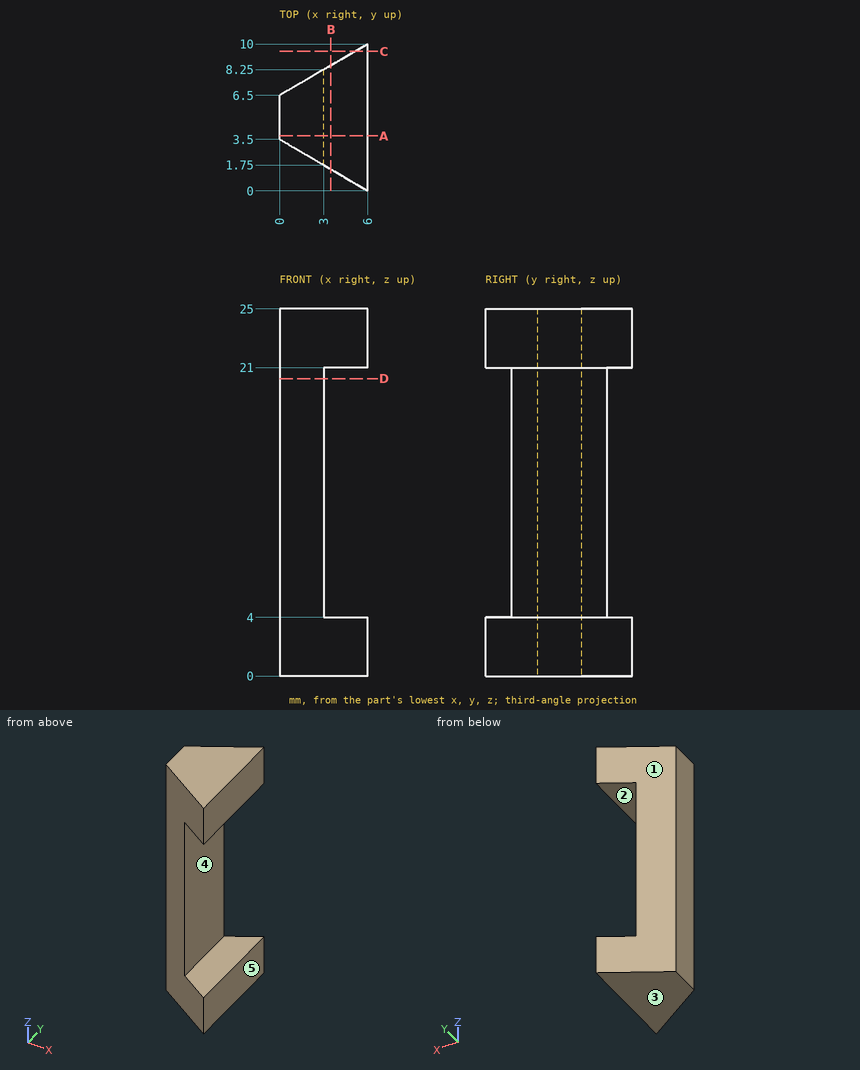
Input: dimensioned drawing with shaded views. Units: mm. Origin: part minimum x, y, z. A direction names the side the tool comes from. Give positions to 0.01 mm unless a question says otherwise; leave off trailing zeros. Write each loop counter-clockwise with the first axis right and the second up, starting at its lowest first coordinate (ties: lowest second). Pieces come first, ordered by that corner, then holes.
1. Section query D-D (z = 20.25). Return the cut outline in (x, y).
2. Pull-direction query (Z, two-part tool) for the marked faces 3, 4 and 5; classes: +Z half, -Z half, draft (parallel to the pull), parting line (faces both ways), or undercut.
3. Section query C-C (y = 9.5). Return the cut outline in (x, z).
4. Section query B-B (x = 3.5). Return the cut outline in (y, z).
5. Material intervals for line 1 along Z through (x, y) = (4, 4.25); line 2 along X through (y, z) = (3.75, 17.5); line 3 along X through (y, z) = (2, 22.75), sorted ascending.
6. First-contact query: pin 1 (1.5 mm diameter, centred on y = 2.5, z = 8, fed in from -X); pin 2 (1 mm diameter, centred on x = 1.5, z = 4, fed in from -Y); pin 3 (5 mm diameter, centred on y = 6.5, z = 13, fed in from +X). Flat tips, straight axial feed; report the tip coordinate or a pass-through.
7. Section query A-A (y = 3.75). Return the cut outline in (x, z), then the cut area to 3 significant figures.
8. Access query for the marked faces 1 and 2. Directions: +Z, -Z, +X, -X, +Y, -Y. A direction counts if a zero-diameter tool reaches every point of the face in a straight line with its end or side. Return the directions, or none.
Output values:
1. outline: (0, 3.5) - (3, 1.75) - (3, 8.25) - (0, 6.5) - close
2. face 3: -Z half
2. face 4: undercut
2. face 5: draft
3. outline: (5.14, 0) - (6, 0) - (6, 4) - (5.14, 4) - close; (5.14, 21) - (6, 21) - (6, 25) - (5.14, 25) - close
4. outline: (1.46, 0) - (8.54, 0) - (8.54, 4) - (1.46, 4) - close; (1.46, 21) - (8.54, 21) - (8.54, 25) - (1.46, 25) - close
5. line 1: z = 0 to 4, 21 to 25
5. line 2: x = 0 to 3
5. line 3: x = 2.57 to 6
6. pin 1: stops at x = 0.43
6. pin 2: stops at y = 2.33
6. pin 3: stops at x = 3
7. outline: (0, 0) - (6, 0) - (6, 4) - (3, 4) - (3, 21) - (6, 21) - (6, 25) - (0, 25) - close
7. area: 99.0 mm2
8. face 1: +Z, -Z, -X, +Y
8. face 2: +X, +Y, -Y
